Input: part model. Units: mm. Frame: model coordinates. A direction names the side the tool comes from. Coordinates: 2 decimals unless noted, no trailing zeros. Write each loop counter-clockwise with the first axis right and the second up, starting at its lowest first coordinate (ties: lowest second). Pieces come first, ordered by that corner, then holes. Notation, with made-up numbers: (65.25, -30.5) - (105.25, -30.5) arc R24 cw to (105.25, -16.5) - close; hole circle Ø8 at (50, 38.5). An arc over 180 degrees is marked (long way). One line per question, with ' | ' between items. Start each with the question number.
1) Section query B-B on z = 0.25. Return loops of the section in (x, y).
2) Reachability of faces 4 (the flat face through (4, 16, 78.75)), 5 (the flat face through (-77.5, 9, 1)), 6 (the cylindrical face through (76.359, 13.064, 89.547)), 7 (the flat face through (77.5, 13, -1)), 8 (the flat face through (-67, 19.2, 1)) from +Z, -Z, +X, -X, +Y, -Y: full face, straight path, thin tool, end or side. Return the list, or none.
3) First-contact query: P1, Ø5, axis at x = -24.5, z = 55, coming from the +Y side; P2, Ø6, axis at x = -52, z = -28.5, coming from the +Y side; P3, Ø23.5, axis at y = 19.5, z = -5.5, coming from the -X side. Flat tips, straight axial feed; report the tip coordinate or a pass-through.
4) Section query D-D on x = -67.5. Return loops of the section in (y, z), and give its area (3 significant figures).
5) Line query: line 1 (Z direction, x = 22, y = 1); line 2 (Z direction, x = 41.5, y = 17.5); line 3 (X direction, y = 20, z = 32.5). Output: solid intervals per line, ascending.
6) Draft query along Z for faces 1 (the cylindrical face through (7.62, 2.46, -11.16)), 2 (the flat face through (-68, 46.5, -73)), 3 (the cylindrical face through (-70.752, 41.43, -87.393)). Return one class per face: released by +Z, released by -Z, zero draft, split by the parting line, or undercut.
7) Section query A-A on x = 22.5. Return loops of the section in (y, z).
8) Section query C-C on y = 15.5. Return loops of the section in (x, z), and give its area (3 significant figures).
Autodesk Inventor part; units mm, degrees
ref_plane "YZ Plane" through (0, 0, 0) normal (1, 0, 0) x (0, 1, 0)
ref_plane "XZ Plane" through (0, 0, 0) normal (0, 1, 0) x (-1, 0, 0)
ref_plane "XY Plane" through (0, 0, 0) normal (0, 0, 1) x (1, 0, 0)
sketch "Skizze1" plane through (0, 0, 0) normal (0, 1, 0) x (-1, 0, 0)
  line L0 (73.5, -90.75) -> (-73.5, -90.75)
  line L1 (-77.5, -86.75) -> (-77.5, 86.75)
  line L2 (-73.5, 90.75) -> (73.5, 90.75)
  line L3 (77.5, 86.75) -> (77.5, -86.75)
  line L4 (77.5, -90.75) -> (-77.5, 90.75) construction
  line L5 (-77.5, -90.75) -> (77.5, 90.75) construction
  arc A0 (77.5, 86.75) -> (73.5, 90.75) centre (73.5, 86.75) ccw
  arc A1 (73.5, -90.75) -> (77.5, -86.75) centre (73.5, -86.75) ccw
  arc A2 (-77.5, -86.75) -> (-73.5, -90.75) centre (-73.5, -86.75) ccw
  arc A3 (-73.5, 90.75) -> (-77.5, 86.75) centre (-73.5, 86.75) ccw
  line L6 (41.5, 78.75) -> (-51.5, 78.75)
  line L7 (-51.5, 78.75) -> (-51.5, -36.75)
  line L8 (-51.5, -36.75) -> (41.5, -36.75)
  line L9 (41.5, -36.75) -> (41.5, 78.75)
  line L10 (41.5, 78.75) -> (-51.5, -36.75) construction
  line L11 (-51.5, 78.75) -> (41.5, -36.75) construction
  point P0 (0, 0)
  point P1 (-5, 21)
  dimension "d0" = 155
  dimension "d1" = 181.5
  dimension "d2" = 4
  dimension "d3" = 12
  dimension "d4" = 26
  dimension "d5" = 54
  dimension "d6" = 36
extrude "Extrusion1" add sketch "Skizze1" along normal blind 26.5
sketch "Skizze2" plane through (0, 0, 0) normal (0, -1, 0) x (1, 0, 0)
  line L0 (-73.5, 90.75) -> (73.5, 90.75)
  arc A0 (-73.5, 90.75) -> (-77.5, 86.75) centre (-73.5, 86.75) ccw
  line L1 (-77.5, -86.75) -> (-77.5, 86.75)
  arc A1 (-77.5, -86.75) -> (-73.5, -90.75) centre (-73.5, -86.75) ccw
  line L2 (73.5, -90.75) -> (-73.5, -90.75)
  arc A2 (73.5, -90.75) -> (77.5, -86.75) centre (73.5, -86.75) ccw
  line L3 (77.5, 86.75) -> (77.5, -86.75)
  arc A3 (77.5, 86.75) -> (73.5, 90.75) centre (73.5, 86.75) ccw
  line L4 (-41.5, 78.75) -> (-41.5, -36.75)
  line L5 (51.5, 78.75) -> (-41.5, 78.75)
  line L6 (51.5, -36.75) -> (51.5, 78.75)
  line L7 (-41.5, -36.75) -> (51.5, -36.75)
  circle A4 centre (22.5, 0.25) radius 18.75
  point P0 (0, 0)
  dimension "d9" = 37.5
  dimension "d11" = 90.5
  dimension "d14" = 55
extrude "Extrusion2" add sketch "Skizze2" against normal blind 5 contours L0 A3 L3 A2 L2 A1 L1 A0 | L5 L6 L7 L4
sketch "Skizze3" plane through (-73.5, 0, 90.75) normal (0, 0, 1) x (1, 0, 0)
  line L0 (-4, 0) -> (-4, 26.5)
  line L1 (0, 0) -> (0, 26.5)
  line L2 (-4, 0) -> (-4, 26.5)
  line L3 (-4, 26.5) -> (16, 26.5)
  line L4 (16, 26.5) -> (16, 19.2)
  line L5 (16, 19.2) -> (-4, 19.2)
  line L6 (-4, 19.2) -> (-4, 26.5)
  point P0 (73.5, 0)
  point P1 (-4, 19.2)
  dimension "d15" = 7.3
  dimension "d16" = 20
extrude "Extrusion3" cut sketch "Skizze3" against normal through all
sketch "Skizze4" plane through (0, 26.5, 0) normal (0, 1, 0) x (1, 0, 0)
  line L0 (-57.5, 90.75) -> (-57.5, -90.75)
  line L1 (-57.5, -90.75) -> (73.5, -90.75)
  arc A0 (73.5, -90.75) -> (77.5, -86.75) centre (73.5, -86.75) ccw
  line L2 (77.5, -86.75) -> (77.5, 86.75)
  arc A1 (77.5, 86.75) -> (73.5, 90.75) centre (73.5, 86.75) ccw
  line L3 (73.5, 90.75) -> (-57.5, 90.75)
  line L4 (-41.5, -78.75) -> (-41.5, 36.75)
  line L5 (-41.5, 36.75) -> (51.5, 36.75)
  line L6 (51.5, 36.75) -> (51.5, -78.75)
  line L7 (51.5, -78.75) -> (-41.5, -78.75)
  arc A2 (-77.5, -86.75) -> (-73.5, -90.75) centre (-73.5, -86.75) ccw
  line L8 (-57.5, -90.75) -> (-73.5, -90.75)
  line L9 (-57.5, -90.75) -> (-57.5, 90.75)
  line L10 (-73.5, 90.75) -> (-57.5, 90.75)
  arc A3 (-73.5, 90.75) -> (-77.5, 86.75) centre (-73.5, 86.75) ccw
  line L11 (-77.5, -86.75) -> (-77.5, 86.75)
  circle A4 centre (-67.5, 72.75) radius 22.5
  point P0 (0, 0)
  dimension "d19" = 45
  dimension "d20" = 10
  dimension "d21" = 18
extrude "Extrusion4" add sketch "Skizze4" along normal blind 10 contours L3 A4 L0 | L10 A3 L11 A4 L3 | L0 A4 L11 A3 L10
sketch "Skizze5" plane through (-67.5, 36.5, -72.75) normal (0, 1, 0) x (1, 0, 0)
  circle A0 centre (0, 0) radius 22.5
  circle A1 centre (0, 0) radius 15
  point P0 (67.5, -72.75)
  dimension "d24" = 30
extrude "Extrusion5" add sketch "Skizze5" along normal blind 10 contours A1
equation "\"Biegeradius\" = Stärke"
equation "\"BreiteBiegungsfreistellung\" = Stärke"
equation "\"TiefeBiegungsfreistellung\" = 0.5 * Stärke"
equation "\"GrößeEckenfreistellung\" = 4 * Stärke"
equation "\"MinimalRest\" = 2 * Stärke"
equation "\"Übergangsradius\" = Biegeradius"
equation "\"JacobiRadiusGröße\" = Biegeradius"
equation "\"Abstandsgröße\" = Stärke"
properties part number "00_XYTable_china_75_55mm"
Answer key:
1) outline: (-77.5, 0) - (3.75, 0) - (3.75, 5) - (-41.5, 5) - (-41.5, 26.5) - (-57.5, 26.5) - (-57.5, 19.2) - (-77.5, 19.2) - close; (41.25, 0) - (77.5, 0) - (77.5, 26.5) - (51.5, 26.5) - (51.5, 5) - (41.25, 5) - close
2) face 4: +Y | face 5: +Z, -Z, -X, -Y | face 6: +Z, +X, +Y, -Y | face 7: +Z, -Z, +X, +Y, -Y | face 8: +Z, -Z, -X
3) P1: y = 5 | P2: y = 26.5 | P3: x = -77.5
4) outline: (0, -90.75) - (19.2, -90.75) - (19.2, 90.75) - (0, 90.75) - close; (26.5, -95.25) - (36.5, -95.25) - (36.5, -87.75) - (46.5, -87.75) - (46.5, -57.75) - (36.5, -57.75) - (36.5, -50.25) - (26.5, -50.25) - close | area: 4,230 mm²
5) line 1: -90.75 to -18.49, 18.99 to 90.75 | line 2: -90.75 to -36.75, 78.75 to 90.75 | line 3: -57.5 to -41.5, 51.5 to 77.5
6) face 1: undercut | face 2: zero draft | face 3: split by the parting line
7) outline: (0, -90.75) - (26.5, -90.75) - (26.5, -36.75) - (5, -36.75) - (5, -18.5) - (0, -18.5) - close; (0, 19) - (5, 19) - (5, 78.75) - (26.5, 78.75) - (26.5, 90.75) - (0, 90.75) - close
8) outline: (-77.5, -86.75) arc R4 ccw to (-73.5, -90.75) - (73.5, -90.75) arc R4 ccw to (77.5, -86.75) - (77.5, 86.75) arc R4 ccw to (73.5, 90.75) - (-73.5, 90.75) arc R4 ccw to (-77.5, 86.75) - close; hole (-41.5, -36.75) - (51.5, -36.75) - (51.5, 78.75) - (-41.5, 78.75) - close | area: 17,400 mm²
